```python
from build123d import *

# Parameters (mm, degrees)
T_LE_DE_BASE_PLI_E1_DEPTH = 10
ENL_V_MAT_EXTRU_1_DEPTH   = 405.598566483
ESQUISSE7_R               = 16
ENL_V_MAT_EXTRU_2_DEPTH   = 10


# Sheet-metal steps are written as plain solids
with BuildPart() as part:
    # Esquisse1 → Tôle de base pliée1 (new body)
    with BuildSketch(Plane.XY):
        Polygon((0, 0), (-60, 400), (60, 400), align=None)
    extrude(amount=-T_LE_DE_BASE_PLI_E1_DEPTH)

    # Esquisse6 → Enlèv. mat.-Extru.1 (cut, through all)
    with BuildSketch(Plane(origin=(0, 0, -10), x_dir=(-1, 0, 0), z_dir=(0, 0, -1))):
        Polygon((60, 400), (0, 400), (54.297112843, 361.980752285), align=None)
        Polygon((-54.297112843, 361.980752285), (0, 400), (-60, 400), align=None)
    extrude(amount=-ENL_V_MAT_EXTRU_1_DEPTH, mode=Mode.SUBTRACT)

    # Esquisse7 → Enlèv. mat.-Extru.2 (cut)
    with BuildSketch(Plane(origin=(0, 0, -10), x_dir=(-1, 0, 0), z_dir=(0, 0, -1))):
        with Locations((0, 335)):
            Circle(ESQUISSE7_R)
    extrude(amount=-ENL_V_MAT_EXTRU_2_DEPTH, mode=Mode.SUBTRACT)


solid = part.part
```
Read the model definition and answer for the solid it produces. Units are mm, in the model's axes. Give positions to 0.01 mm unless a question says otherwise; leave off trailing zeros. Order: outer loops, then holes, each group sorted by start corner. A loop starts at its lowest first (then second) coordinate and runs counter-clockwise, first axis right, second up.
(1) Find section C-C (z = -7). Give the vertices of the cut face in (x, y), plus the area to 3 significant figures.
(2) Find section D-D (y = 249). Give the vertices of the cut face in (x, z).
(3) Find section A-A (y = 335). Give the vertices of the cut face in (x, z).
(4) Find section B-B (x = -11.5). Give the vertices of the cut face in (y, z).
(5) Straight lines are drawn through the part: L1, parallel to X at y = 92, z = -2.75; L2, parallel to X at y = 341, z = -5; L3, parallel to X at y = 175, z = -9.5. For each, find the intervals that lie inside material, in ascending order.
(6) Given pin 1 (5 mm diameter, centred on y = 43.5, z = -2, fed in from -X); pin 2 (4 mm diameter, centred on y = 211.5, z = -1, fed in from +X) (3 decimals); pin 3 (6 mm diameter, centred on y = 312.5, z = -3.5, fed in from +X) (3 decimals), each flat-ended and moving along its own axis, determine where each tip first touches the part or whether it passes through.
(7) For a pull along Y with two mould halves and no side action, classify faces 1 (the flat face through (27.53, 183.52, -4.93)), 2 (the flat face through (1, 247, 0)), 3 (the cylindrical face through (3.47, 319.38, -5.07)), 4 (the flat face through (27.529, 380.724, -5.07)) as released by +Y, released by -Y, zero draft, split by the parting line, or undercut.
Result sheet:
1. outline: (-54.3, 361.98) - (0, 0) - (54.3, 361.98) - (0, 400) - close; hole circle Ø32 at (0, 335)
1. area: 20,900 mm2
2. outline: (-37.35, -10) - (37.35, -10) - (37.35, 0) - (-37.35, 0) - close
3. outline: (-50.25, -10) - (-16, -10) - (-16, 0) - (-50.25, 0) - close; (16, -10) - (50.25, -10) - (50.25, 0) - (16, 0) - close
4. outline: (76.67, -10) - (323.88, -10) - (323.88, 0) - (76.67, 0) - close; (346.12, -10) - (391.95, -10) - (391.95, 0) - (346.12, 0) - close
5. L1: x = -13.8 to 13.8
5. L2: x = -51.15 to -14.83, 14.83 to 51.15
5. L3: x = -26.25 to 26.25
6. pin 1: stops at x = -6.9
6. pin 2: stops at x = 32.025
6. pin 3: stops at x = 47.325
7. face 1: released by -Y
7. face 2: zero draft
7. face 3: undercut
7. face 4: released by +Y
